Check sheet for the modelled part. Datum: model origin and axes. Units: mm. A direction names the side the tool comes from. Round coordinates to 2 decimals unless told otherwise and drop trailing zeros. Write each loop counter-clockwise with the first axis right and the second up, starting at its lowest first coordinate (ties: lowest second). Pieces come first, ordered by that corner, then holes.
Item 1: Cross-section at B-B on x = -13.5. Enter the section's corners in (y, z).
Item 2: Tool access check on faces 1 (the flat face through (-12.91, 835.72, 1.13)), 2 (the cylindrical face through (42.4, 866.4, 1.1)). Record the directions out of +Z, -Z, +X, -X, +Y, -Y that give a thin tool (end or side, any length) a straight path to the whole face; none if there is none.
Item 3: Material ranges on line 1 (Y direction, x = -7, z = 0.3); line 2 (X direction, y = 693.5, z = 2.15); line 3 (Y direction, x = -43, z = 0.95), recorded low to high.
Item 4: Cross-section at A-A on x = 19. Enter the section's corners in (y, z).
Item 5: Release check for a two-part mould opening along Y. For faces 3 (the cylindrical face through (36.708, 781.357, 1.127)), 4 (the cylindrical face through (-31.652, 680.168, 1.127)), 5 (the cylindrical face through (6.81, 896.97, 1.13)), 6 (the cylindrical face through (68.96, 671.346, 1.127)) record: +Y half, -Y half, draft (parallel to the pull), parting line (faces both ways), or undercut.
Item 6: Cross-section at C-C on z = 0.45. Count the separate pieces of the cut face and the enclosed holes in it, plus the area to 3 significant figures.
Item 7: Go/stop test with flat-tipped pins: pin 1 Ø4.5 at (x, y) = (57.79, 847.7) entering from +Z; pin 2 Ø0.7 at (y, z) = (752.5, 1.5) entering from -X. Record where each tip stops, or that it passes through.
from build123d import *

# Parameters (mm, degrees)
SKETCH1_R           = 2.4892
SKETCH1_R_2         = 2.37186857
BOSS_EXTRUDE2_DEPTH = 2.286


with BuildPart() as part:
    # Sketch1 → Boss-Extrude2 (new body)
    with BuildSketch(Plane.XY):
        with BuildLine():
            Line((65.40759274, 898.497727162), (48.89759274, 898.497727162))
            ThreePointArc((48.89759274, 898.497727162), (45.305490291, 897.009829611), (43.81759274, 893.417727162))
            Line((43.81759274, 893.417727162), (43.81759274, 869.922727162))
            ThreePointArc((43.81759274, 869.922727162), (42.329695188, 866.330624714), (38.73759274, 864.842727162))
            Line((38.73759274, 864.842727162), (13.33759274, 864.842727162))
            ThreePointArc((13.33759274, 864.842727162), (9.745490291, 866.330624714), (8.25759274, 869.922727162))
            Line((8.25759274, 869.922727162), (8.25759274, 893.417727162))
            ThreePointArc((8.25759274, 893.417727162), (6.769695188, 897.009829611), (3.17759274, 898.497727162))
            Line((3.17759274, 898.497727162), (-56.51240726, 898.497727162))
            ThreePointArc((-56.51240726, 898.497727162), (-60.104509709, 897.009829611), (-61.59240726, 893.417727162))
            Line((-61.59240726, 893.417727162), (-61.59240726, 875.096507696))
            ThreePointArc((-61.59240726, 875.096507696), (-61.239653123, 873.236522064), (-60.230381059, 871.634850458))
            Line((-60.230381059, 871.634850458), (-11.051271068, 818.81429954))
            ThreePointArc((-11.051271068, 818.81429954), (2.568990945, 784.197727162), (-11.051271068, 749.581154784))
            Line((-11.051271068, 749.581154784), (-60.230381059, 696.760603866))
            ThreePointArc((-60.230381059, 696.760603866), (-61.239653123, 695.15893226), (-61.59240726, 693.298946628))
            Line((-61.59240726, 693.298946628), (-61.59240726, 674.977727162))
            ThreePointArc((-61.59240726, 674.977727162), (-60.104509709, 671.385624714), (-56.51240726, 669.897727162))
            Line((-56.51240726, 669.897727162), (3.17759274, 669.897727162))
            ThreePointArc((3.17759274, 669.897727162), (6.769695188, 671.385624714), (8.25759274, 674.977727162))
            Line((8.25759274, 674.977727162), (8.25759274, 698.472727162))
            ThreePointArc((8.25759274, 698.472727162), (9.745490291, 702.064829611), (13.33759274, 703.552727162))
            Line((13.33759274, 703.552727162), (38.73759274, 703.552727162))
            ThreePointArc((38.73759274, 703.552727162), (42.329695188, 702.064829611), (43.81759274, 698.472727162))
            Line((43.81759274, 698.472727162), (43.81759274, 674.977727162))
            ThreePointArc((43.81759274, 674.977727162), (45.305490291, 671.385624714), (48.89759274, 669.897727162))
            Line((48.89759274, 669.897727162), (65.40759274, 669.897727162))
            ThreePointArc((65.40759274, 669.897727162), (68.999695188, 671.385624714), (70.48759274, 674.977727162))
            Line((70.48759274, 674.977727162), (70.48759274, 784.197727162))
            Line((70.48759274, 784.197727162), (70.48759274, 893.417727162))
            ThreePointArc((70.48759274, 893.417727162), (68.999695188, 897.009829611), (65.40759274, 898.497727162))
        make_face()
        with Locations((-31.11240726, 885.797727162)):
            Circle(SKETCH1_R, mode=Mode.SUBTRACT)
        with Locations((-18.41240726, 885.797727162)):
            Circle(SKETCH1_R, mode=Mode.SUBTRACT)
        with Locations((-5.71240726, 885.797727162)):
            Circle(SKETCH1_R, mode=Mode.SUBTRACT)
        with Locations((57.78759274, 860.397727162)):
            Circle(SKETCH1_R_2, mode=Mode.SUBTRACT)
        with Locations((57.78759274, 847.697727162)):
            Circle(SKETCH1_R, mode=Mode.SUBTRACT)
        with Locations((57.78759274, 834.997727162)):
            Circle(SKETCH1_R, mode=Mode.SUBTRACT)
        with Locations((57.78759274, 822.297727162)):
            Circle(SKETCH1_R, mode=Mode.SUBTRACT)
        with Locations((57.78759274, 809.597727162)):
            Circle(SKETCH1_R, mode=Mode.SUBTRACT)
        with Locations((-5.71240726, 682.597727162)):
            Circle(SKETCH1_R, mode=Mode.SUBTRACT)
        with Locations((-18.41240726, 682.597727162)):
            Circle(SKETCH1_R, mode=Mode.SUBTRACT)
        with Locations((-31.11240726, 682.597727162)):
            Circle(SKETCH1_R, mode=Mode.SUBTRACT)
        with Locations((57.78759274, 733.397727162)):
            Circle(SKETCH1_R, mode=Mode.SUBTRACT)
        with Locations((57.78759274, 720.697727162)):
            Circle(SKETCH1_R, mode=Mode.SUBTRACT)
        with Locations((57.78759274, 707.997727162)):
            Circle(SKETCH1_R, mode=Mode.SUBTRACT)
        with Locations((57.78759274, 682.597727162)):
            Circle(SKETCH1_R, mode=Mode.SUBTRACT)
        with Locations((57.78759274, 885.797727162)):
            Circle(SKETCH1_R, mode=Mode.SUBTRACT)
        with Locations((57.78759274, 771.497727162)):
            Circle(SKETCH1_R, mode=Mode.SUBTRACT)
        with Locations((57.78759274, 758.797727162)):
            Circle(SKETCH1_R, mode=Mode.SUBTRACT)
        with Locations((57.78759274, 746.097727162)):
            Circle(SKETCH1_R, mode=Mode.SUBTRACT)
        with Locations((-56.51240726, 885.797727162)):
            Circle(SKETCH1_R, mode=Mode.SUBTRACT)
        with Locations((-43.81240726, 885.797727162)):
            Circle(SKETCH1_R, mode=Mode.SUBTRACT)
        with Locations((-43.81240726, 682.597727162)):
            Circle(SKETCH1_R, mode=Mode.SUBTRACT)
        with Locations((-56.51240726, 682.597727162)):
            Circle(SKETCH1_R, mode=Mode.SUBTRACT)
        with Locations((57.78759274, 796.897727162)):
            Circle(SKETCH1_R, mode=Mode.SUBTRACT)
        with Locations((57.78759274, 784.197727162)):
            Circle(SKETCH1_R, mode=Mode.SUBTRACT)
        with Locations((57.78759274, 873.097727162)):
            Circle(SKETCH1_R_2, mode=Mode.SUBTRACT)
        with Locations((57.78759274, 695.297727162)):
            Circle(SKETCH1_R, mode=Mode.SUBTRACT)
        with BuildLine():
            Line((-22.612168162, 846.141069924), (-2.925323721, 824.996523604))
            ThreePointArc((-2.925323721, 824.996523604), (0.611406899, 823.381415049), (4.254307315, 824.740207043))
            Line((4.254307315, 824.740207043), (26.964490273, 845.884753363))
            ThreePointArc((26.964490273, 845.884753363), (28.230078898, 851.462712794), (23.502833035, 854.682727162))
            Line((23.502833035, 854.682727162), (-18.894194364, 854.682727162))
            ThreePointArc((-18.894194364, 854.682727162), (-23.552070423, 851.630186315), (-22.612168162, 846.141069924))
        make_face(mode=Mode.SUBTRACT)
        with BuildLine():
            Line((40.00759274, 791.795734585), (40.00759274, 839.416910928))
            ThreePointArc((40.00759274, 839.416910928), (36.955051892, 844.074786987), (31.465935502, 843.134884727))
            Line((31.465935502, 843.134884727), (7.715964553, 821.022233244))
            ThreePointArc((7.715964553, 821.022233244), (6.100855998, 817.485502624), (7.459647992, 813.842602208))
            Line((7.459647992, 813.842602208), (31.209618941, 788.334077347))
            ThreePointArc((31.209618941, 788.334077347), (36.787578372, 787.068488722), (40.00759274, 791.795734585))
        make_face(mode=Mode.SUBTRACT)
        with BuildLine():
            Line((7.459647992, 754.552852117), (31.209618941, 780.061376977))
            ThreePointArc((31.209618941, 780.061376977), (36.787578372, 781.326965602), (40.00759274, 776.599719739))
            Line((40.00759274, 776.599719739), (40.00759274, 728.978543396))
            ThreePointArc((40.00759274, 728.978543396), (36.955051892, 724.320667337), (31.465935502, 725.260569598))
            Line((31.465935502, 725.260569598), (7.715964553, 747.37322108))
            ThreePointArc((7.715964553, 747.37322108), (6.100855998, 750.909951701), (7.459647992, 754.552852117))
        make_face(mode=Mode.SUBTRACT)
        with BuildLine():
            Line((26.964490273, 722.510700961), (4.254307315, 743.655247282))
            ThreePointArc((4.254307315, 743.655247282), (0.611406899, 745.014039275), (-2.925323721, 743.398930721))
            Line((-2.925323721, 743.398930721), (-22.612168162, 722.2543844))
            ThreePointArc((-22.612168162, 722.2543844), (-23.552070423, 716.765268009), (-18.894194364, 713.712727162))
            Line((-18.894194364, 713.712727162), (23.502833035, 713.712727162))
            ThreePointArc((23.502833035, 713.712727162), (28.230078898, 716.93274153), (26.964490273, 722.510700961))
        make_face(mode=Mode.SUBTRACT)
    extrude(amount=BOSS_EXTRUDE2_DEPTH)


solid = part.part
Response values:
1. outline: (669.9, 0) - (713.71, 0) - (713.71, 2.29) - (669.9, 2.29) - close; (732.04, 0) - (746.95, 0) - (746.95, 2.29) - (732.04, 2.29) - close; (821.44, 0) - (836.35, 0) - (836.35, 2.29) - (821.44, 2.29) - close; (854.68, 0) - (898.5, 0) - (898.5, 2.29) - (854.68, 2.29) - close
2. face 1: +Z, -Z
2. face 2: +Z, -Z, +Y
3. line 1: y = 669.9 to 680.47, 684.73 to 713.71, 739.02 to 754.52, 813.87 to 829.37, 854.68 to 883.67, 887.93 to 898.5
3. line 2: x = -61.59 to 8.26, 43.82 to 56.07, 59.51 to 70.49
3. line 3: y = 669.9 to 680.24, 684.95 to 715.27, 853.13 to 883.44, 888.15 to 898.5
4. outline: (703.55, 0) - (713.71, 0) - (713.71, 2.29) - (703.55, 2.29) - close; (729.93, 0) - (736.87, 0) - (736.87, 2.29) - (729.93, 2.29) - close; (766.95, 0) - (801.45, 0) - (801.45, 2.29) - (766.95, 2.29) - close; (831.53, 0) - (838.47, 0) - (838.47, 2.29) - (831.53, 2.29) - close; (854.68, 0) - (864.84, 0) - (864.84, 2.29) - (854.68, 2.29) - close
5. face 3: undercut
5. face 4: undercut
5. face 5: +Y half
5. face 6: -Y half
6. separate pieces: 1
6. enclosed holes: 31
6. area: 15,800 mm2
7. pin 1: passes through
7. pin 2: stops at x = -8.82
